Could you check a few things on this model? Use its own coordinates, in mm. Face numbers are marked on the shaded views. Give positions to 0.01 mm unless a question says otherwise; leave off trailing zeros. Loops run counter-clockwise (first coordinate to the right, second up) from the corner with the lowest first, then second, coordinate; pieces in that order, holes last. Notation, with made-up numbers: M -31.75,-2 L -19.75,-2 A7 cw -19.75,11 Z; hole C 89.25,25 d3. An arc over 180 degrees is marked long. Use a Markdown table: item, result. Add a question column.
1) Suppose I cut it at A-A on x = -315.5. List the corners of the cut face in (y, z) for me, and give its area (3 significant figures).
2) Suppose I cut it at C-C on y = -59.5. List the corners of the cut face in (x, z) for me, and give its area (3 significant figures).
3) Will these pins go through, and if not, where does the flat tip stop? pin 1 Ø4 at (x, y) = (-327.5, -60) entering from +Z; pin 2 Ø12 at (x, z) = (-377.5, 59) entering from -Y; pin 3 Ø6 at (x, z) = (-336.5, 130) entering from -Y; pin 4 Ø8 at (x, y) = (-317.5, -67) entering from +Z.
4) If I drill on line 1 along X through (y, z) = (-69, 136.5); line 2 along Y through (x, z) = (-350.5, 27); line 3 along Z through (x, y) = (-338, -80.5), over which ranges is the centre line in solid material (lowest first)? Write a range as [from, to].
5) We'd pull the mould along Z, two halves only. Please class the marked faces 1, 2 and 3: +Z half, -Z half, draft (parallel to the pull), parting line (faces both ways), or undercut.
6) Suppose I cut it at B-B on z = 91. List the corners of the cut face in (x, y) for me.
```python
from build123d import *

# Parameters (mm, degrees)
F0_W      = 445
F0_H      = 100
F1_DEPTH  = 1000
F2_ANGLE  = -5
F3_ANGLE  = -120
F5_ANGLE  = -120
F8_ANGLE  = -120
F10_ANGLE = -120
F12_ANGLE = -120
F14_W     = 401.3673663139
F14_H     = 945.5828145146
F15_DEPTH = 33
F17_SCALE = 0.2


with BuildPart() as f1:
    # F0 (on Top) → F1 (new body)
    with BuildSketch(Plane.XY):
        with Locations((-164.5579262078, -35.3550005704)):
            Rectangle(F0_W, F0_H)
    extrude(amount=F1_DEPTH)


with BuildPart() as f1_1:
    # F2: moved
    add(f1.part.rotate(Axis((-164.5579262078, 14.6449994296, 0), (1, 0, 0)), F2_ANGLE))


with BuildPart() as f3_1:
    # F3: copy of F1
    add(f1_1.part.rotate(Axis((57.9420737922, -41.3965990058, 506.8129233206), (0, -0.0871557427, -0.9961946981)), F3_ANGLE))


with BuildPart() as f3_1_1:
    # F4: moved
    add(f3_1.part.moved(Location((87, 55, 0))))


with BuildPart() as f5_1:
    # F5: copy of F3_1
    add(f3_1_1.part.rotate(Axis((280.8395334138, -420.1211463803, 544.7589043088), (0, -0.0871557427, -0.9961946981)), F5_ANGLE))


with BuildPart() as f5_1_1:
    # F6: moved
    add(f5_1.part.moved(Location((91, -75, 0))))


with BuildPart() as f3_1_2:
    # F7: moved
    add(f3_1_1.part.moved(Location((13, -17, 0))))


with BuildPart() as f8_1:
    # F8: copy of F5_1
    add(f5_1_1.part.rotate(Axis((62.7369930353, -829.2262239457, 573.9893110223), (0, -0.0871557427, -0.9961946981)), F8_ANGLE))


with BuildPart() as f8_1_1:
    # F9: moved
    add(f8_1.part.moved(Location((-17, -111, 0))))


with BuildPart() as f10_1:
    # F10: copy of F8_1
    add(f8_1_1.part.rotate(Axis((-399.2630069647, -840.6067541365, 565.2737367476), (0, -0.0871557427, -0.9961946981)), F10_ANGLE))


with BuildPart() as f10_1_1:
    # F11: moved
    add(f10_1.part.moved(Location((-104, -42, 0))))


with BuildPart() as f12_1:
    # F12: copy of F10_1
    add(f10_1_1.part.rotate(Axis((-639.1604665862, -448.8822067619, 527.3277557595), (0, -0.0871557427, -0.9961946981)), F12_ANGLE))


with BuildPart() as f12_1_1:
    # F13: moved
    add(f12_1.part.moved(Location((-65, 57, 0))))


with BuildPart() as f1_2:
    add(f1_1.part)

    # F14 (on face) → F15 (cut)
    with BuildSketch(Plane(origin=(0, -85.0857156038, 7.4440355433), x_dir=(1, 0, 0), z_dir=(0, -0.9961946981, 0.0871557427))):
        with Locations((-162.8310680389, 495.9846995771)):
            Rectangle(F14_W, F14_H)
    extrude(amount=-F15_DEPTH, mode=Mode.SUBTRACT)


with BuildPart() as f1_3:
    # F17: moved
    add(f1_2.part.scale(F17_SCALE).moved(Location((-309.6463409662, -67.9795763037, 6.9724594198))))


solid = f1_3.part
```
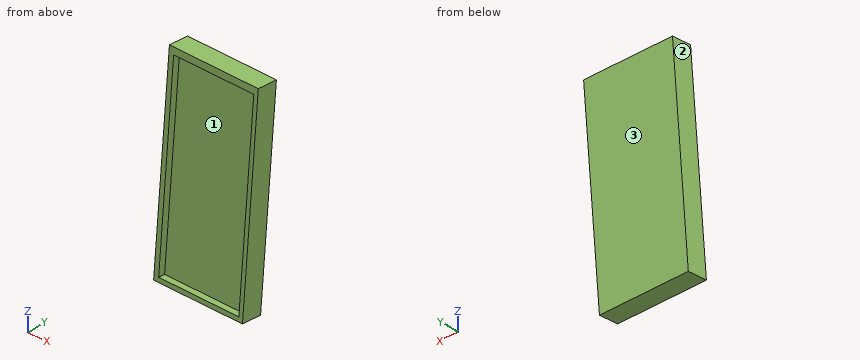
Answer block:
| question | item | result |
|---|---|---|
| 1 | outline | M -84.97,8.72 L -65.05,6.97 L -47.62,206.21 L -67.54,207.95 L -68.11,201.48 L -61.53,200.9 L -78.02,12.51 L -84.59,13.08 Z |
| 1 | area | 2,750 mm^2 |
| 2 | outline | M -387.06,70.42 L -298.06,70.42 L -298.06,207.25 L -387.06,207.25 Z |
| 2 | area | 12,200 mm^2 |
| 3 | pin 1 | stops at z = 207.47 |
| 3 | pin 2 | stops at y = -80.88 |
| 3 | pin 3 | stops at y = -68 |
| 3 | pin 4 | stops at z = 207.95 |
| 4 | line 1 | x = [-387.06, -382.35], [-302.08, -298.06] |
| 4 | line 2 | y = [-76.75, -63.3] |
| 4 | line 3 | z = [8.32, 12.72] |
| 5 | face 1 | undercut |
| 5 | face 2 | draft |
| 5 | face 3 | -Z half |
| 6 | outline | M -387.06,-77.78 L -382.35,-77.78 L -382.35,-71.15 L -302.08,-71.15 L -302.08,-77.78 L -298.06,-77.78 L -298.06,-57.7 L -387.06,-57.7 Z |
